from build123d import *

# Parameters (mm, degrees)
F0_R     = 1.65
F0_W     = 5
F0_H     = 36.5884533238
F0_H_2   = 27.6073180421
F0_W_2   = 4.2823543772
F0_H_3   = 20.4163840114
F1_DEPTH = 5.08


# Not quite as in the source:
# - a feature names something its author has since deleted; it is built from what else it names


with BuildPart() as f1:
    # F0 (on Top) → F1 (new body)
    with BuildSketch(Plane.XY):
        Polygon((21.25, 36.8060796608), (-21.25, 36.8060796608), (-42.5, 0), (-21.25, -36.8060796608), (-14.481, -36.8060796608), (-9.481, -36.8060796608), (-9.481, -29.0118510268), (-16.75, -29.0118510268), (-25.125, -14.5059255134), (-27.6471267629, -10.137473817), (-33.5, 0), (-23.128253194, 17.9643924312), (-20.4351344929, 22.6290108523), (-16.75, 29.0118510268), (-2.0468940441, 29.0118510268), (2.2354603331, 29.0118510268), (16.75, 29.0118510268), (19.1722516141, 24.8163881624), (21.9975489559, 19.92282962), (33.5, 0), (27.7069725582, -10.0338178588), (25.125, -14.5059255134), (16.75, -29.0118510268), (8.019, -29.0118510268), (8.019, -36.8060796608), (13.019, -36.8060796608), (21.25, -36.8060796608), (42.5, 0), align=None)
        with Locations((-18.75, -32.4759526419)):
            Circle(F0_R, mode=Mode.SUBTRACT)
        with Locations((18.75, -32.4759526419)):
            Circle(F0_R, mode=Mode.SUBTRACT)
        with Locations((-37.5, 0)):
            Circle(F0_R, mode=Mode.SUBTRACT)
        with Locations((-18.75, 32.4759526419)):
            Circle(F0_R, mode=Mode.SUBTRACT)
        with Locations((37.5, 0)):
            Circle(F0_R, mode=Mode.SUBTRACT)
        with Locations((18.75, 32.4759526419)):
            Circle(F0_R, mode=Mode.SUBTRACT)
        with Locations((-11.981, -55.1003063227)):
            Rectangle(F0_W, F0_H)
        with Locations((10.519, -55.1003063227)):
            Rectangle(F0_W, F0_H)
        Polygon((-9.481, -73.3945329846), (-14.481, -73.3945329846), (-14.481, -83.3945329846), (13.019, -83.3945329846), (13.019, -73.3945329846), (8.019, -73.3945329846), (7.019, -73.3945329846), (4.8774445356, -73.3945329846), (-6.1735640291, -73.3945329846), (-8.481, -73.3945329846), align=None)
        with BuildLine():
            ThreePointArc((-7.831, -78.3945329846), (-10.647726189, -79.5612591736), (-9.481, -76.7445329846))
            ThreePointArc((-9.481, -76.7445329846), (-8.314273811, -77.2278067957), (-7.831, -78.3945329846))
        make_face(mode=Mode.SUBTRACT)
        with BuildLine():
            ThreePointArc((9.669, -78.3945329846), (6.852273811, -79.5612591736), (8.019, -76.7445329846))
            ThreePointArc((8.019, -76.7445329846), (9.185726189, -77.2278067957), (9.669, -78.3945329846))
        make_face(mode=Mode.SUBTRACT)
        Polygon((-6.3394445356, -36.8060796608), (-8.481, -36.8060796608), (-8.481, -40.8093024077), (-2.6512739295, -55.0297430961), (-0.7737012417, -50.3825876202), align=None)
        Polygon((7.019, -40.7417911932), (7.019, -36.8060796608), (4.7115640291, -36.8060796608), (-0.7737012417, -50.3825876202), (1.1892739295, -55.1708695493), align=None)
        with Locations((-0.002691932, -15.2081920057)):
            Rectangle(F0_W, F0_H_2)
        Polygon((-9.481, -1.4045329846), (-9.481, -2.4605728254), (-8.1094596477, -1.4045329846), align=None)
        Polygon((-8.481, -69.4588214522), (-8.481, -73.3945329846), (-6.1735640291, -73.3945329846), (-0.6882987583, -59.8180250252), (-2.6512739295, -55.0297430961), align=None)
        Polygon((4.8774445356, -73.3945329846), (7.019, -73.3945329846), (7.019, -69.3913102377), (1.1892739295, -55.1708695493), (-0.6882987583, -59.8180250252), align=None)
        Polygon((2.497308068, -1.4045329846), (8.019, -1.4045329846), (11.781800831, -1.4045329846), (13.019, -1.4045329846), (13.019, 4.3879779564), (13.019, 5.6842228109), (13.019, 8.5954670154), (8.9436992999, 8.5954670154), (2.2354603331, 8.5954670154), (-2.0468940441, 8.5954670154), (-9.4036843662, 8.5954670154), (-14.481, 8.5954670154), (-14.481, 6.9638797721), (-14.481, 0), (-14.481, -1.4045329846), (-9.481, -1.4045329846), (-8.1094596477, -1.4045329846), (-2.502691932, -1.4045329846), align=None)
        with BuildLine():
            ThreePointArc((-7.831, 3.5954670154), (-8.314273811, 2.4287408264), (-9.481, 1.9454670154))
            ThreePointArc((-9.481, 1.9454670154), (-10.647726189, 4.7621932043), (-7.831, 3.5954670154))
        make_face(mode=Mode.SUBTRACT)
        with BuildLine():
            ThreePointArc((9.669, 3.5954670154), (9.185726189, 2.4287408264), (8.019, 1.9454670154))
            ThreePointArc((8.019, 1.9454670154), (6.852273811, 4.7621932043), (9.669, 3.5954670154))
        make_face(mode=Mode.SUBTRACT)
        Polygon((1.1892739295, -55.1708695493), (-0.7737012417, -50.3825876202), (-2.6512739295, -55.0297430961), (-0.6882987583, -59.8180250252), align=None)
        Polygon((11.781800831, -1.4045329846), (25.125, -14.5059255134), (27.7069725582, -10.0338178588), (13.019, 4.3879779564), (13.019, -1.4045329846), align=None)
        Polygon((-20.4351344929, 22.6290108523), (-23.128253194, 17.9643924312), (-14.481, 6.9638797721), (-14.481, 8.5954670154), (-9.4036843662, 8.5954670154), align=None)
        Polygon((13.019, 5.6842228109), (21.9975489559, 19.92282962), (19.1722516141, 24.8163881624), (8.9436992999, 8.5954670154), (13.019, 8.5954670154), align=None)
        with Locations((0.0942831445, 18.8036590211)):
            Rectangle(F0_W_2, F0_H_3)
    extrude(amount=F1_DEPTH)


solid = f1.part
Design review of the part built by this model. Coordinates are the model's own, in mm. Round coordinates to 2 decimals unless told otherwise and drop trailing zeros. Write each loop counter-clockwise with the first axis right and the second up, starting at its lowest first coordinate (ties: lowest second). Pieces come first, ordered by that corner, then holes. Notation, with made-up numbers: (9.25, 87.5) -> (65.25, 87.5) arc R30 ccw to (65.25, 109.5) -> close; hole circle Ø7 at (77, 73). An arc over 180 degrees is marked (long way). One line per item, written item: value. Start each with the question number.
Q1. Add section A-A (x = 37.5). Give the boundary of the cut face in (y, z).
Q2. The part is to be moulded in two halves that separate along Y. For faces 1 (the face through (-32.02, -18.15, 2.5)), 2 (the face through (7.019, -39, 3)), say which applies: pulls with the +Y half, pulls with the -Y half, needs draft (parallel to the pull), parting line crosses it, or undercut.
Q3. Add section B-B (y = -11.5). Give the boundary of the cut face in (x, z).
Q4. Add section C-C (y = 15.5). Give the boundary of the cut face in (x, z), then the cut area to 3 significant figures.
Q5. Add section D-D (z = 2.3). State how many separate pieces and enclosed holes the cut face has, then the cut area to 3 significant figures.
Q6. To check wall thickness, follow probe 1 along X at (y, z) = (-70, 4.4); probe 2 along X at (y, z) = (31, 0.35); probe 3 along X at (y, z) = (-42, 1.45). State the ranges of each line that lie inside material, in increasing order.
Q7. Insertion check: P1, Ø3, axis at x = -22.5, z = 1, coming from the -Y side; P2, Ø3, axis at y = -39, z = 2, coming from the +X side; P3, Ø1.5, axis at y = -51.5, z = 1.5, coming from the -X side. Each pin has a flat end and moves straight along its axis. Give the tip position at first contact, or say it passes through.
Response:
1. outline: (-8.66, 0) -> (-1.65, 0) -> (-1.65, 5.08) -> (-8.66, 5.08) -> close; (1.65, 0) -> (8.66, 0) -> (8.66, 5.08) -> (1.65, 5.08) -> close
2. face 1: pulls with the -Y half
2. face 2: undercut
3. outline: (-35.86, 0) -> (-26.86, 0) -> (-26.86, 5.08) -> (-35.86, 5.08) -> close; (-2.5, 0) -> (2.5, 0) -> (2.5, 5.08) -> (-2.5, 5.08) -> close; (22.06, 0) -> (35.86, 0) -> (35.86, 5.08) -> (22.06, 5.08) -> close
4. outline: (-33.55, 0) -> (-24.55, 0) -> (-24.55, 5.08) -> (-33.55, 5.08) -> close; (-21.19, 0) -> (-14.83, 0) -> (-14.83, 5.08) -> (-21.19, 5.08) -> close; (-2.05, 0) -> (2.24, 0) -> (2.24, 5.08) -> (-2.05, 5.08) -> close; (13.3, 0) -> (19.21, 0) -> (19.21, 5.08) -> (13.3, 5.08) -> close; (24.55, 0) -> (33.55, 0) -> (33.55, 5.08) -> (24.55, 5.08) -> close
4. area: 176 mm^2
5. separate pieces: 1
5. enclosed holes: 15
5. area: 3,200 mm^2
6. probe 1: x = -14.48 to -9.48, -8.48 to -4.8, 3.49 to 7.02, 8.02 to 13.02
6. probe 2: x = -24.6 to -19.49, -18.01 to 18.01, 19.49 to 24.6
6. probe 3: x = -14.48 to -9.48, -7.99 to -4.21, 2.61 to 6.51, 8.02 to 13.02
7. P1: stops at y = -36.81
7. P2: stops at x = 13.02
7. P3: stops at x = -14.48
